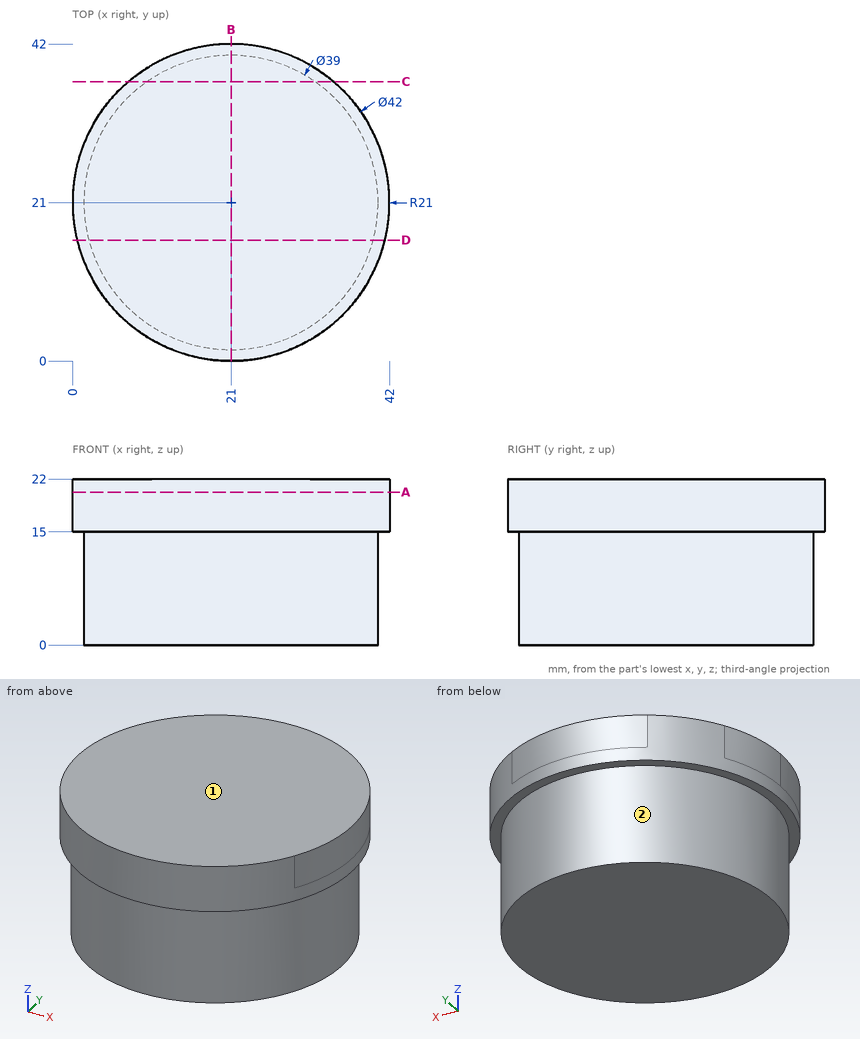
Here's the drawing with two shaded views (mm, measured from the low corner). I have some questions. A direction names the side the tool comes from. Coordinates: 2 decimals unless noted, no trailing zeros. Loops run counter-clockwise (first coordinate to the right, second up) from the corner with the lowest first, then second, coordinate; pieces in that order, holes last. Notation, with made-up numbers: (39.5, 53) -> (73.5, 53) arc R25 ccw to (73.5, 73) -> close; hole circle Ø4 at (-12, 45). An arc over 180 degrees is marked (long way). Answer as a JSON object with one key per item and string values.
1) Imagine slicing it at C-C (y = 37). Please give me the cut outline in (x, z).
Results:
{"outline": "(7.4, 15) -> (9.85, 15) -> (9.85, 0) -> (32.15, 0) -> (32.15, 15) -> (34.6, 15) -> (34.6, 22) -> (7.4, 22) -> close"}
2) For the marked faces 1 and 2, which set-ups out of +Z, -Z, +X, -X, +Y, -Y let a thin tool reach every point of the face, with its end or its side?
Results:
{"face 1": "+Z, +X, -X, +Y, -Y", "face 2": "-Z"}
3) For P1, Ø1, axis at x = 32.5, y = 32.5, coming from the -Z side; P2, Ø1.5, axis at x = 19, z = 17.5, coming from the +Y side; P3, Ø4, axis at y = 18, z = 3, coming from the +X side; P4, Ø5, axis at x = 9, z = 17.5, coming from the -Y side, each with a flat end and sliding along its axis, tell me the tip position at first contact or that it passes through.
Results:
{"P1": "stops at z = 0", "P2": "stops at y = 41.96", "P3": "stops at x = 40.47", "P4": "stops at y = 2.27"}
4) Imagine slicing it at B-B (x = 21). Please give me the cut outline in (y, z).
Results:
{"outline": "(0, 15) -> (1.5, 15) -> (1.5, 0) -> (40.5, 0) -> (40.5, 15) -> (42, 15) -> (42, 22) -> (0, 22) -> close"}
5) Imagine slicing it at A-A (z = 20.25). Please give me the cut outline in (x, y).
Results:
{"outline": "(0, 21) arc R21 ccw to (2.81, 10.5) arc R21 ccw to (39.19, 10.5) arc R21 ccw to (39.19, 31.5) arc R21 ccw to (31.5, 39.19) arc R21 ccw to (10.5, 39.19) arc R21 ccw to (2.81, 31.5) arc R21 ccw to start"}
6) Imagine slicing it at D-D (y = 16). Please give me the cut outline in (x, z), then the cut area to 3 significant figures.
Results:
{"outline": "(0.6, 15) -> (2.15, 15) -> (2.15, 0) -> (39.85, 0) -> (39.85, 15) -> (41.4, 15) -> (41.4, 22) -> (0.6, 22) -> close", "area": "851 mm^2"}
7) If I drill on line 1 (Z direction, x = 6.5, y = 7); line 2 (X direction, y = 21.5, z = 2.5); line 3 (X direction, y = 8, z = 5), over which ranges is the centre line in solid material (lowest first)?
Results:
{"line 1": "z = 15 to 22", "line 2": "x = 1.51 to 40.49", "line 3": "x = 6.47 to 35.53"}
